```python
from build123d import *

# Parameters (mm, degrees)
SKETCH1_W                                         = 65.532
SKETCH1_H                                         = 82.55
EXTRUDE1_DEPTH                                    = 3.175
CSK_FOR_2_FLAT_HEAD_MACHINE_SCREW_100_D           = 2.4384
CSK_FOR_2_FLAT_HEAD_MACHINE_SCREW_100_CSINK_D     = 4.3688
CSK_FOR_2_FLAT_HEAD_MACHINE_SCREW_100_CSINK_ANGLE = 100
SKETCH3_W                                         = 22.225
SKETCH3_H                                         = 12.7
CUT_EXTRUDE1_DEPTH                                = 4.175
TAP_DRILL_FOR_2_TAP1_D                            = 1.778
TAP_DRILL_FOR_2_TAP1_DEPTH                        = 6.35
TAP_DRILL_FOR_2_TAP1_TIP                          = 0.53416509


with BuildPart() as part:
    # Sketch1 → Extrude1 (new body)
    with BuildSketch(Plane(origin=(0, 0, 0), x_dir=(1, 0, 0), z_dir=(0, 1, 0))):
        with Locations((0, 7.9375)):
            Rectangle(SKETCH1_W, SKETCH1_H)
    extrude(amount=EXTRUDE1_DEPTH)

    # CSK for #2 Flat Head Machine Screw (100)1 (through all)
    with Locations(Plane(origin=(-26.416, 3.175, 31.75), x_dir=(0, 0, 1), z_dir=(0, 1, 0))):
        with Locations((0, 0), (0, 52.832), (-52.387499988, -4.7625), (-11.1125, -4.7625), (-52.3875, 57.5945), (-11.1125, 57.5945)):
            CounterSinkHole(CSK_FOR_2_FLAT_HEAD_MACHINE_SCREW_100_D / 2, CSK_FOR_2_FLAT_HEAD_MACHINE_SCREW_100_CSINK_D / 2, counter_sink_angle=CSK_FOR_2_FLAT_HEAD_MACHINE_SCREW_100_CSINK_ANGLE)

    # Sketch3 → Cut-Extrude1 (cut, through all)
    with BuildSketch(Plane(origin=(0, 3.175, 0), x_dir=(-1, 0, 0), z_dir=(0, 1, 0))):
        with Locations((-21.6535, -42.8625)):
            Rectangle(SKETCH3_W, SKETCH3_H)
    extrude(amount=-CUT_EXTRUDE1_DEPTH, mode=Mode.SUBTRACT)

    # Tap Drill for #2 Tap1
    with Locations(Plane(origin=(24.638, 0, -17.0815), x_dir=(0, 0, -1), z_dir=(0, -1, 0))):
        with Locations((0, 0), (-1.905, -50.038), (-37.084, -49.784), (-44.069, 1.524)):
            Hole(TAP_DRILL_FOR_2_TAP1_D / 2, depth=TAP_DRILL_FOR_2_TAP1_DEPTH)
            with Locations((0, 0, -(TAP_DRILL_FOR_2_TAP1_DEPTH + TAP_DRILL_FOR_2_TAP1_TIP / 2))):  # 118° drill point
                Cone(0, TAP_DRILL_FOR_2_TAP1_D / 2, TAP_DRILL_FOR_2_TAP1_TIP, mode=Mode.SUBTRACT)


solid = part.part
```
Work out the finished part from the listing and answer in its coordinate system (mm). Round coordinates to 2 decimals unless told otherwise and drop trailing zeros. Write each loop counter-clockwise with the first axis right and the second up, starting at its lowest first coordinate (ties: lowest second). Pieces come first, ordered by that corner, then holes.
1) A cutting plane is placed at C-C on x = 15. Determine the outline of the cut face in (y, z) (1 decimal), and give its area (3 significant figures).
2) A cutting plane is placed at A-A on z = 31.75. Determine the outline of the cut face in (x, y) (3 decimals).
3) Determine the mould class of faces 1 (the face through (29.99, 1.17, -20.37)), 2 (the face through (22, 2, -36.512)), 3 (the face through (-32.766, 2, -7)) for opening direction X: pulls with the +X half, pulls with the -X half, needs draft (parallel to the pull), parting line crosses it, or undercut.
4) Consider probe 1 along X at (y, z) = (1.5, 31.75); probe 2 along Z at (x, y) = (26.5, 1.35); probe 3 along X at (y, z) = (0.9, -40). Determine where each line is inside the solid, lowest interval first.
5) Flat-ended cylindrical pins translate along their axes: P1, Ø2, axis at x = 26.416, z = 31.75, coming from the -Y side; P2, Ø1, axis at x = 23, y = 2, coming from the -Z side. Find the tip coordinate at first contact, or state that the pin passes through.
6) A cutting plane is placed at B-B on y = 0.75. Give the number of separate pieces and of enclosed holes in the cut face, and give its area (3 significant figures).
Entries:
1. outline: (0, -36.5) - (3.2, -36.5) - (3.2, 33.3) - (0, 33.3) - close
1. area: 222 mm2
2. outline: (-32.766, 0) - (-27.635, 0) - (-27.635, 2.365) - (-28.6, 3.175) - (-32.766, 3.175) - close; (-25.197, 0) - (25.197, 0) - (25.197, 2.365) - (24.232, 3.175) - (-24.232, 3.175) - (-25.197, 2.365) - close; (27.635, 0) - (32.766, 0) - (32.766, 3.175) - (28.6, 3.175) - (27.635, 2.365) - close
3. face 1: undercut
3. face 2: needs draft
3. face 3: pulls with the -X half
4. probe 1: x = -32.77 to -27.64, -25.2 to 25.2, 27.64 to 32.77
4. probe 2: z = -36.51 to 26.17, 27.81 to 30.53, 32.97 to 33.34
4. probe 3: x = -32.77 to 10.54
5. P1: passes through
5. P2: stops at z = -36.51
6. separate pieces: 1
6. enclosed holes: 10
6. area: 5,090 mm2
